Here's the drawing with two shaded views (mm, measured from the low corner). I have some questions. Coordinates: 2 decimals unless noted, no trailing zeros. Write each loop counter-clockwise with the first axis right and the second up, starting at its lowest first coordinate (ties: lowest second). Pieces come first, ordered by that corner, then holes.
Item 1: If I drill on line 1 (Y direction, x = 5, z = 2.1); line 2 (Y direction, x = 13, z = 0.9); line 3 (Y direction, x = 15.5, z = 2.25), over which ranges is the centre line in solid material (lowest first)?
Item 2: If we section it at D-D (x = 24.75): Please give me the cut outline in (y, z), then the cut area to 3 significant figures.
Item 3: If we section it at C-C (z = 1.95): Please give me the cut outline in (x, y), then the cut area to 3 significant figures.
Item 4: We'd pull the mould along X, two halves only. Please class the marked faces 1, 2 and 3: +X half, -X half, draft (parallel to the pull), parting line (faces both ways), or undercut.
Item 5: If we section it at A-A (y = 15): Please give me the cut outline in (x, z), then the cut area to 3 significant figures.
Item 6: If we section it at B-B (x = 13): Please give me the cut outline in (y, z).
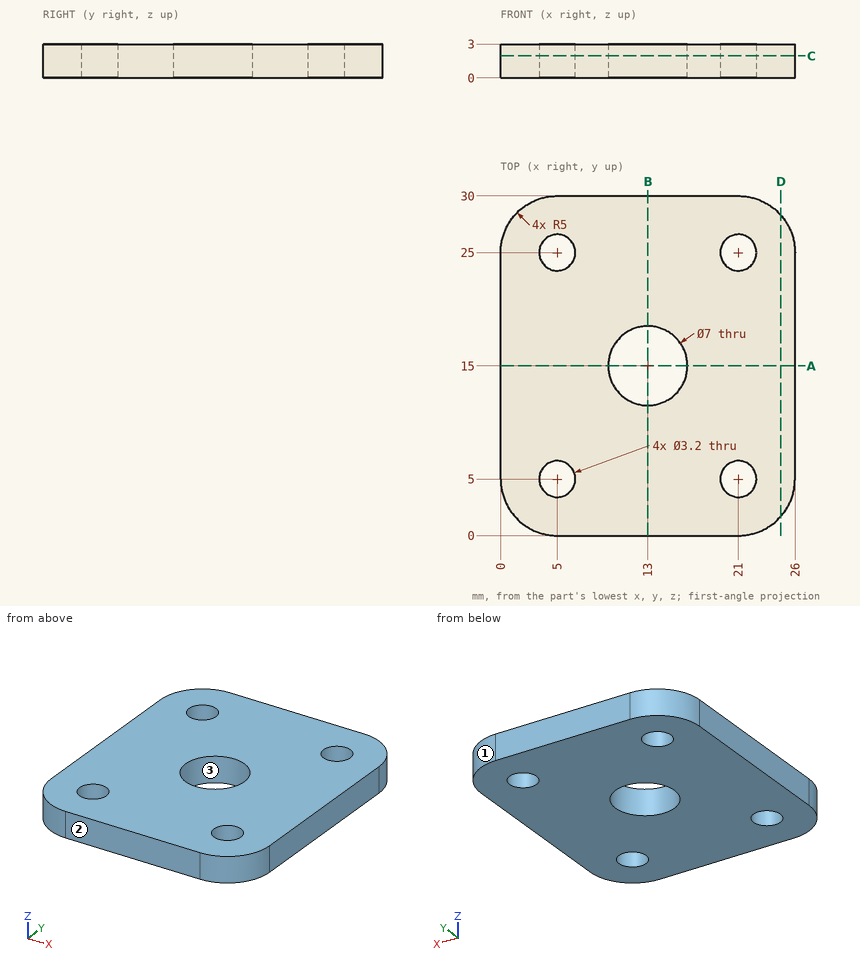
Answer list:
1. line 1: y = 0 to 3.4, 6.6 to 23.4, 26.6 to 30
1. line 2: y = 0 to 11.5, 18.5 to 30
1. line 3: y = 0 to 12.55, 17.45 to 30
2. outline: (1.69, 0) - (28.31, 0) - (28.31, 3) - (1.69, 3) - close
2. area: 79.8 mm2
3. outline: (0, 5) arc R5 ccw to (5, 0) - (21, 0) arc R5 ccw to (26, 5) - (26, 25) arc R5 ccw to (21, 30) - (5, 30) arc R5 ccw to (0, 25) - close; hole circle Ø3.2 at (5, 5); hole circle Ø3.2 at (5, 25); hole circle Ø7 at (13, 15); hole circle Ø3.2 at (21, 5); hole circle Ø3.2 at (21, 25)
3. area: 688 mm2
4. face 1: +X half
4. face 2: draft
4. face 3: undercut
5. outline: (0, 0) - (9.5, 0) - (9.5, 3) - (0, 3) - close; (16.5, 0) - (26, 0) - (26, 3) - (16.5, 3) - close
5. area: 57.0 mm2
6. outline: (0, 0) - (11.5, 0) - (11.5, 3) - (0, 3) - close; (18.5, 0) - (30, 0) - (30, 3) - (18.5, 3) - close
